from build123d import *

# Parameters (mm, degrees)
F0_W     = 6.35
F0_H     = 254
F1_DEPTH = 279.4
F3_DEPTH = 25.4
F4_W     = 79.375
F4_H     = 12.7
F5_DEPTH = 25.4
F7_D     = 6.35


with BuildPart() as f1:
    # F0 (on Front) → F1 (new body)
    with BuildSketch(Plane.XZ):
        Rectangle(F0_W, F0_H)
    extrude(amount=F1_DEPTH)

    # F2 (on face) → F3 (cut)
    with BuildSketch(Plane(origin=(-3.175, 0, 0), x_dir=(0, -1, 0), z_dir=(-1, 0, 0))):
        with BuildLine():
            Line((0, 103.006612), (22.465272, 103.006612))
            Line((22.465272, 103.006612), (174.625, 47.625))
            Line((174.625, 47.625), (12.7, 47.625))
            ThreePointArc((12.7, 47.625), (60.126734, -66.873266), (174.625, -114.3))
            Line((174.625, -114.3), (279.4, -114.3))
            Line((279.4, -114.3), (279.4, 127))
            Line((279.4, 127), (0, 127))
            Line((0, 127), (0, 103.006612))
        make_face()
        with BuildLine():
            Line((174.625, 47.625), (22.465272, 103.006612))
            ThreePointArc((22.465272, 103.006612), (15.160005, 75.742981), (12.7, 47.625))
            Line((12.7, 47.625), (174.625, 47.625))
        make_face()
    extrude(amount=-F3_DEPTH, mode=Mode.SUBTRACT)

    # F4 (on face) → F5 (cut)
    with BuildSketch(Plane(origin=(-3.175, 0, 0), x_dir=(0, -1, 0), z_dir=(-1, 0, 0))):
        with Locations((239.7125, -120.65)):
            Rectangle(F4_W, F4_H)
    extrude(amount=-F5_DEPTH, mode=Mode.SUBTRACT)

    # F7 (through all)
    with Locations(Plane.YZ.offset(3.175)):
        with Locations((-9.525, 93.357041), (-9.525, 0), (-41.275, -73.351197), (-111.125, -114.3), (-182.245, -120.65)):
            Hole(F7_D / 2)


solid = f1.part
For this review, take the finished solid that the model builds, in its own axes (mm). A direction names the side the tool comes from. Round coordinates to 2 decimals unless told otherwise and drop trailing zeros. Loops run counter-clockwise (first coordinate to the right, second up) from the corner with the lowest first, then second, coordinate; pieces in that order, holes last. Notation, with made-up numbers: (63, 26.5) - (105, 26.5) arc R24 ccw to (105, 49.5) - close; hole circle Ø10 at (68.5, -8). An arc over 180 degrees is marked (long way). Put each result on its own line as item: value. Start each with the question number.
1. For faces 4 (the cylindrical face through (-0.044, -58.875, -65.607)), 5 (the flat face through (0, -187, -114.3)), 6 (the flat face through (0, -200.025, -121)), list the 3-axis set-ups (+Z, -Z, +X, -X, +Y, -Y) from which the entire face can be reached by the end or side of a thin tool; tool diameter is ignored.
2. Insertion check: P1, Ø3, axis at x = -1.5, z = -30.5, coming from the +Y side; P2, Ø5.5, axis at y = -111.125, z = -114.3, coming from the +X side; P3, Ø3, axis at x = -2, z = 6, coming from the -Y side. Each pin has a flat end and moves straight along its axis. Give the tip position at first contact, or say it passes through.
3. Consider section B-B on x = -0.75. State the section outline as (y, z) points (3 decimals).
4. Mouldability with a two-part tool opening along Y and no side actions: class faces 1 (the cylindrical face through (-0.044, -114.058, -115.516)), 2 (the flat face through (0, 0, -10)), 3 (the cylindrical face through (-0.04, -15.23, 76.13)) as +Y half, -Y half, draft (parallel to the pull), parting line (faces both ways), or undercut.
5. Consider section A-A on z = -120.65. State the section outline as (x, y) points (3 decimals).
6. For probe 1 along Z at (x, y) = (0.5, -182); probe 2 along Z at (x, y) = (1, -12); probe 3 along Z at (x, y) = (-0.75, -11), list the stretches that pass through material, from the lowest coordinate up. Write a range as [from, to].
7. Consider section D-D on y = -58. State the section outline as (x, z) points (3 decimals).
8. Consider section C-C on z = 0. State the section outline as (x, y) points (3 decimals).
Result sheet:
1. face 4: +X, -X, -Y
1. face 5: +Z, +X, -X, -Y
1. face 6: +Z, -Z, +X, -X, -Y
2. P1: y = 0
2. P2: through
2. P3: y = -18.55
3. outline: (-200.025, -127) - (0, -127) - (0, 103.007) - (-22.465, 103.007) arc R161.925 cw to (-12.7, 47.625) arc R161.925 cw to (-174.625, -114.3) - (-200.025, -114.3) - close; hole circle Ø6.35 at (-182.245, -120.65); hole circle Ø6.35 at (-111.125, -114.3); hole circle Ø6.35 at (-41.275, -73.351); hole circle Ø6.35 at (-9.525, 0); hole circle Ø6.35 at (-9.525, 93.357)
4. face 1: undercut
4. face 2: +Y half
4. face 3: -Y half
5. outline: (-3.175, -200.025) - (3.175, -200.025) - (3.175, -185.42) - (-3.175, -185.42) - close; (-3.175, -179.07) - (3.175, -179.07) - (3.175, 0) - (-3.175, 0) - close
6. probe 1: [-127, -123.82], [-117.48, -114.3]
6. probe 2: [-127, -1.99], [1.99, 91.37], [95.35, 103.01]
6. probe 3: [-127, -2.81], [2.81, 90.55], [96.17, 103.01]
7. outline: (-3.175, -127) - (3.175, -127) - (3.175, -64.706) - (-3.175, -64.706) - close
8. outline: (-3.175, -19.862) - (3.175, -19.862) - (3.175, -12.7) - (-3.175, -12.7) - close; (-3.175, -6.35) - (3.175, -6.35) - (3.175, 0) - (-3.175, 0) - close
